Part model, mm, in its own coordinate system. A direction names the side the tool comes from. Round coordinates to 2 decimals unless told otherwise and drop trailing zeros. Write each loop counter-clockwise with the first axis right and the second up, starting at its lowest first coordinate (ties: lowest second). Pieces come first, ordered by that corner, then holes. Notation, with made-up numbers: M 65.25,-12 L 101.25,-12 A28 ccw 101.25,7 Z; hole C 23,17 d6. An arc over 180 degrees is marked long. Answer as a JSON object with one key per item and string values. Group by question number.
1. Band-saw the part on C-C, the plane z = 1.25. Write the cut outline in (x, y).
2. Which spindle directions (+Z, -Z, +X, -X, +Y, -Y) get a long thin tool onto all of the face, cutting with end or side? Do faces 1 (the face through (2, -4, 0)), 2 (the face through (-1.19, -5.37, 0.99)). Say none if no direction does.
3. Drop flat-ended pins along their axis: pin 1 (1.5 mm diameter, centred on x = 4, z = -1, fed in from -Y); pin 2 (1 mm diameter, centred on y = 4, z = 0.5, fed in from +X); pin 3 (1.5 mm diameter, centred on y = -4.5, z = -5.5, fed in from +X); pin 4 (6.5 mm diameter, centred on x = 0, y = 0, fed in from -Z). Give the stop position or say it passes through.
4. Band-saw the part on D-D, the plane x = -3.75. Write the cut outline in (y, z), plus the area to 3 significant figures.
5. Band-saw the part on A-A, the plane y = 0. Write the cut outline in (x, z), plus the area to 4 significant figures.
6. Drill centre lines: line 1 (Y direction, x = 0, z = 0.7); line 2 (Y direction, x = 0, z = -1.5); line 3 (X direction, y = 2.25, z = -5.5). Where is each one in solid material? Low to high. Write a range as from..to.
from build123d import *

# Parameters (mm, degrees)
F0_R     = 5.5
F0_R_2   = 4.25
F0_R_3   = 3.5
F1_DEPTH = 2
F2_DEPTH = 7.5


# Not quite as in the source:
# - a feature names something its author has since deleted; it is built from what else it names


with BuildPart() as f1:
    # F0 (on Top) → F1 (new body)
    with BuildSketch(Plane.XY):
        Circle(F0_R)
        Circle(F0_R_2, mode=Mode.SUBTRACT)
        Circle(F0_R_2)
        Circle(F0_R_3, mode=Mode.SUBTRACT)
    extrude(amount=F1_DEPTH)

    # F0 (on Top) → F2 (join)
    with BuildSketch(Plane.XY):
        Circle(F0_R_2)
        Circle(F0_R_3, mode=Mode.SUBTRACT)
    extrude(amount=-F2_DEPTH)


solid = f1.part
Worked answers:
{
 "1": {"outline": "C 0,0 d11; hole C 0,0 d7"},
 "2": {"face 1": "-Z", "face 2": "+Z, -Z"},
 "3": {"pin 1": "stops at y = -2.74", "pin 2": "stops at x = 4.24", "pin 3": "stops at x = 2", "pin 4": "passes through"},
 "4": {"outline": "M -4.02,0 L -2,0 L -2,-7.5 L 2,-7.5 L 2,0 L 4.02,0 L 4.02,2 L -4.02,2 Z", "area": "46.1 mm^2"},
 "5": {"outline": "M -5.5,0 L -4.25,0 L -4.25,-7.5 L -3.5,-7.5 L -3.5,2 L -5.5,2 Z; M 3.5,-7.5 L 4.25,-7.5 L 4.25,0 L 5.5,0 L 5.5,2 L 3.5,2 Z", "area": "19.25 mm^2"},
 "6": {"line 1": "y = -5.5..-3.5, 3.5..5.5", "line 2": "y = -4.25..-3.5, 3.5..4.25", "line 3": "x = -3.61..-2.68, 2.68..3.61"}
}
